from build123d import *

# Parameters (mm, degrees)
F1_DEPTH = 63.5
F2_W     = 50.8
F2_H     = 35.000445
F3_DEPTH = 19.051
F4_R     = 1.5875
F5_DEPTH = 63.501


with BuildPart() as f1:
    # F0 (on Front) → F1 (new body)
    with BuildSketch(Plane.XZ):
        with BuildLine():
            Line((-9.525, 6.35), (-9.525, 0))
            Line((-9.525, 0), (-3.082892, -26.15921))
            ThreePointArc((-3.082892, -26.15921), (0, -28.575), (3.082892, -26.15921))
            Line((3.082892, -26.15921), (9.525, 0))
            Line((9.525, 0), (9.525, 6.35))
            Line((9.525, 6.35), (-9.525, 6.35))
        make_face()
    extrude(amount=F1_DEPTH)

    # F2 (on face) → F3 (cut, through all)
    with BuildSketch(Plane.YZ.offset(9.525)):
        with Locations((-31.75, -17.500222)):
            Rectangle(F2_W, F2_H)
    extrude(amount=-F3_DEPTH, mode=Mode.SUBTRACT)

    # F4 (on face) → F5 (cut, through all)
    with BuildSketch(Plane(origin=(0, 0, 0), x_dir=(-1, 0, 0), z_dir=(0, 1, 0))):
        with Locations((0, -25.4)):
            Circle(F4_R)
    extrude(amount=-F5_DEPTH, mode=Mode.SUBTRACT)


solid = f1.part
For this review, take the finished solid that the model builds, in its own axes (mm). A direction names the side the tool comes from. Give positions to 0.01 mm unless a question says otherwise; leave off trailing zeros. Write each loop counter-clockwise with the first axis right and the second up, starting at its lowest first coordinate (ties: lowest second). Pieces come first, ordered by that corner, then holes. Notation, with made-up numbers: (17.25, -37) -> (24.25, -37) arc R20 ccw to (24.25, -12) -> close; hole circle Ø2 at (68.25, 29.25). An arc over 180 degrees is marked (long way). Use CSV: the item, a comma, the result in double quotes.
Q1. To check wall thickness, follow probe 1 along Y at (x, z) = (0.5, -8); probe 2 along Z at (x, y) = (0.75, -6); probe 3 along X at (y, z) = (-3, -25). State the ranges of each line that lie inside material, in increasing order. Write a range as [from, to].
Conclusion:
probe 1,"[-63.5, -57.15], [-6.35, 0]"
probe 2,"[-28.49, -26.8], [-24, 6.35]"
probe 3,"[-3.37, -1.54], [1.54, 3.37]"
Q2. Take a section at A-A, the plane x = 0. State how many separate pieces and enclosed holes the cut face has, then the cut area to 3 significant figures.
Conclusion:
separate pieces,"3"
enclosed holes,"0"
area,"726 mm2"
Q3. Tool access review of faces 1 (the face through (-0.85, -3.13, -24.06)), 2 (the face through (0, -6.35, -11)): name each direction out of +Z, -Z, +X, -X, +Y, -Y from which nothing blocks a thin tool from reaching the whole face with its end or side.
Conclusion:
face 1,"+Y, -Y"
face 2,"-Z, +X, -X"
Q4. Take a section at B-B, the plane z = -25.4. Write out the cut boundary in (x, y).
Conclusion:
outline,"(-3.27, -63.5) -> (-1.59, -63.5) -> (-1.59, -57.15) -> (-3.27, -57.15) -> close; (-3.27, -6.35) -> (-1.59, -6.35) -> (-1.59, 0) -> (-3.27, 0) -> close; (1.59, -63.5) -> (3.27, -63.5) -> (3.27, -57.15) -> (1.59, -57.15) -> close; (1.59, -6.35) -> (3.27, -6.35) -> (3.27, 0) -> (1.59, 0) -> close"
Q5. Take a section at C-C, the plane x = -5.5. Write out the cut boundary in (y, z), then the cut area to 3 significant figures.
Conclusion:
outline,"(-63.5, -16.34) -> (-57.15, -16.34) -> (-57.15, 0) -> (-6.35, 0) -> (-6.35, -16.34) -> (0, -16.34) -> (0, 6.35) -> (-63.5, 6.35) -> close"
area,"611 mm2"
Q6. Mouldability with a two-part tool opening along Z and no side actions: class faces 3 (the face through (0, -32, 0)), 4 (the face through (-0.85, -60.28, -24.06)), 5 (the face through (0, -57.15, -11)) as pulls with the +Z half, pulls with the -Z half, needs draft (parallel to the pull), parting line crosses it, or undercut.
Conclusion:
face 3,"pulls with the -Z half"
face 4,"undercut"
face 5,"needs draft"
Q7. Take a section at D-D, the plane y = -10.5. Write out the cut boundary in (x, z) (3 decimals), then the cut area to 3 significant figures.
Conclusion:
outline,"(-9.525, 0) -> (9.525, 0) -> (9.525, 6.35) -> (-9.525, 6.35) -> close"
area,"121 mm2"
Q8. For P1, Ø5.5, axis at x = -0.5, y = -41.5, coming from the -Z side; P2, Ø5, axis at x = -3.5, z = -22.5, coming from the +Y side; P3, Ø4, axis at y = -11.5, z = -3.5, coming from the -X side, all flat-tipped, find the tip position at first contact; note any pin that passes through.
Conclusion:
P1,"z = 0"
P2,"y = 0"
P3,"through"
